Design review of the part built by this model. Coordinates are the model's own, in mm. A direction names the side the tool comes from. Round coordinates to 2 decimals unless told otherwise and drop trailing zeros. Write each loop counter-clockwise with the first axis right and the second up, starting at its lowest first coordinate (ties: lowest second). Pieces come first, ordered by that corner, then holes. Notation, with made-up numbers: M 79,-29 L 114,-29 A26 ccw 114,0 Z; hole C 19,47.5 d1. An arc over 180 degrees is marked long. Use CSV: the item, a comma, the result in double quotes.
Autodesk Inventor part; units mm, degrees
ref_plane "YZ Plane" through (0, 0, 0) normal (1, 0, 0) x (0, 1, 0)
ref_plane "XZ Plane" through (0, 0, 0) normal (0, 1, 0) x (-1, 0, 0)
ref_plane "XY Plane" through (0, 0, 0) normal (0, 0, 1) x (1, 0, 0)
sketch "Boceto1" plane through (0, 0, 0) normal (0, 0, 1) x (1, 0, 0)
  point P0 (0, 0)
sketch "Boceto2" plane through (0, 0, 0) normal (0, 1, 0) x (-1, 0, 0)
  line L0 (0, 0) -> (104, 0)
  line L1 (250, -30) -> (250, -90)
  line L2 (104, -120) -> (0, -120)
  arc A0 (100, -90) -> (100, -30) centre (100, -60) ccw
  line L3 (250, -60) -> (250, -30)
  arc A1 (155.9615, -30) -> (104, 0) centre (104, -60) ccw
  arc A2 (104, -120) -> (155.9615, -90) centre (104, -60) ccw
  line L4 (0, -120) -> (0, -90)
  line L5 (0, -30) -> (0, 0)
  line L6 (0, -90) -> (100, -90)
  line L7 (155.9615, -90) -> (250, -90)
  line L8 (250, -30) -> (155.9615, -30)
  line L9 (100, -30) -> (0, -30)
  dimension "d2" = 60
  dimension "d3" = 150
  dimension "d4" = 4
extrude "Extrusión1" add sketch "Boceto2" along normal blind 100
sketch "Boceto3" plane through (-104, 0, 0) normal (0, 0, 1) x (1, 0, 0)
  arc A0 (17.3394, 16) -> (17.3394, 84) centre (54, 50) ccw
  line L0 (0, 100) -> (104, 100)
  line L1 (104, 0) -> (104, 100)
  line L2 (0, 0) -> (104, 0)
  circle A1 centre (54, 50) radius 25
  line L3 (-146, 80) -> (8.1742, 80)
  line L4 (8.1742, 20) -> (-146, 20)
  arc A2 (17.3394, 16) -> (8.1742, 20) centre (8.1742, 7.5) ccw
  arc A3 (8.1742, 80) -> (17.3394, 84) centre (8.1742, 92.5) ccw
  line L5 (-146, 80) -> (-146, 20)
  line L6 (-146, 0) -> (-146, 100)
  line L7 (-146, 0) -> (-51.9615, 0)
  line L8 (-146, 100) -> (-51.9615, 100)
  dimension "d7" = 50
  dimension "d9" = 25
  dimension "d10" = 25
  dimension "d11" = 60
  dimension "d12" = 20
  dimension "d13" = 20
extrude "Extrusión2" cut sketch "Boceto3" against normal blind 200 contours A2 L4 L5 L3 A3 A0 keep common part
sketch "Boceto4" plane through (-250, 20, -30) normal (-1, 0, 0) x (0, 0, 1)
  line L0 (-60, 60) -> (0, 60)
  line L1 (0, 60) -> (-17.4, 60)
  line L2 (0, 60) -> (0, 42.6)
  line L3 (0, 0) -> (0, 60)
  line L4 (0, 42.6) -> (-17.4, 60)
  line L5 (-42.6, 60) -> (-60, 42.6)
  line L6 (-60, 60) -> (-60, 42.6)
  line L7 (-60, 60) -> (-42.6, 60)
  line L8 (-60, 17.4) -> (-42.6, 0)
  line L9 (-60, 0) -> (-42.6, 0)
  line L10 (-60, 0) -> (-60, 17.4)
  line L11 (-17.4, 0) -> (0, 17.4)
  line L12 (0, 0) -> (0, 17.4)
  line L13 (0, 0) -> (-17.4, 0)
  point P0 (30, -20)
  point P1 (-30, 30)
  dimension "d16" = 17.4
  dimension "d17" = 17.4
  dimension "d20" = 360
extrude "Extrusión3" cut sketch "Boceto4" against normal blind 60
sketch "Boceto6" plane through (-250, 37.4, -30) normal (-1, 0, 0) x (0, 0, 1)
  circle A0 centre (-30, 12.6) radius 25
  line L0 (0, 0) -> (0, 25.2)
  line L1 (-17.4, -17.4) -> (-42.6, -17.4)
  point P0 (30, -37.4)
  dimension "d24" = 50
  dimension "d25" = 30
  dimension "d26" = 30
fillet "Empalme1" radius 12 4 edges at (-190, 71.3, -38.7) (-190, 71.3, -81.3) (-190, 28.7, -81.3) (-190, 28.7, -38.7)
extrude "Extrusión4" add sketch "Boceto6" along normal blind 150.7
properties part number "Fork end" material "Plástico PC/ABS"
1) Wall thickness on line 1 along Y through (x, z) = (-50, -21.5); line 2 along Z through (x, y) = (-35.5, 12.5); line 3 along X through (y, z) = (28.5, -18.5): over which ranges is each line inside the solid? List them lowest first. Write a range as [from, to].
Answers:
line 1,"[0, 25], [75, 100]"
line 2,"[-120, -90], [-30, 0]"
line 3,"[-147.33, -62.76], [-37.24, -4.86]"
2) The part is to be moulded in two halves that separate along X. For faces 1 (the face through (-157, 80, -59)), 2 (the face through (-70, 35, -105)), 3 (the face through (-195.009, 27.233, -36.99)), 4 (the face through (-0.03, 48.32, -104.79)), say which applies: released by +X, released by -X, zero draft, split by the parting line, or undercut.
Answers:
face 1,"zero draft"
face 2,"undercut"
face 3,"released by -X"
face 4,"split by the parting line"
3) Add section C-C on z = -60. Write out the cut boundary in (x, y).
Answers:
outline,"M -400.7,25 L -250,25 L -250,20 L -130,20 L -130,80 L -250,80 L -250,75 L -400.7,75 Z"
4) Add section D-D on y = 12. Write out the cut boundary in (x, z).
Answers:
outline,"M -82.5,-120 L -17.5,-120 L -17.5,-90 L -82.5,-90 Z; M -82.5,-30 L -17.5,-30 L -17.5,0 L -82.5,0 Z"
5) Add section B-B on x = -50. Write out the cut boundary in (y, z), then the cut area to 3 significant figures.
Answers:
outline,"M 0,-120 L 25,-120 L 25,-90 L 0,-90 Z; M 0,-30 L 25,-30 L 25,0 L 0,0 Z; M 75,-120 L 100,-120 L 100,-90 L 75,-90 Z; M 75,-30 L 100,-30 L 100,0 L 75,0 Z"
area,"3,000 mm²"
6) Add section A-A on y = 50. Write out the cut boundary in (x, z).
Answers:
outline,"M -400.7,-85 L -250,-85 L -250,-90 L -155.96,-90 A60 ccw -104,-120 L -75,-120 L -75,-90 L -100,-90 A30 cw -100,-30 L -75,-30 L -75,0 L -104,0 A60 ccw -155.96,-30 L -250,-30 L -250,-35 L -400.7,-35 Z; M -25,-120 L 0,-120 L 0,-90 L -25,-90 Z; M -25,-30 L 0,-30 L 0,0 L -25,0 Z"
7) Machinability: for faces 5 (the face through (-193, 50, -30)), 6 (the face through (-324, 65, -80)), 7 (the face through (-192, 50, -90)), 8 (the face through (-72.9, 60.4, -30)), which of the approach directions +Z, -Z, +X, -X, +Y, -Y give a long, thin tool a straight path to every point of the face, cutting with its end or side? Answer none if there is none.
Answers:
face 5,"+Z, -X, +Y, -Y"
face 6,"-X"
face 7,"-Z, -X, +Y, -Y"
face 8,"+X, +Y, -Y"
8) For pin 1 Ø6 at (y, z) = (64, -23.5) entering from -X; pin 2 Ø8 at (x, z) = (-343.5, -38) entering from +Y; pin 3 Ø12 at (y, z) = (20, -68) entering from -X, all flat-tipped, find the tip position at first contact; note any pin that passes through.
Answers:
pin 1,"x = -153.78"
pin 2,"y = 67.35"
pin 3,"x = -250"
